Verification items for the finished model (mm, model axes). Round coordinates to 2 decimals unless told otherwise and drop trailing zeros. Order: outer loops, then holes, each group sorted by start corner. A loop starts at its lowest first (then second) coordinate and runs counter-clockwise, first axis right, second up. Notation, with made-up numbers: (20, 51.5) -> (35, 51.5) arc R23 cw to (35, 80.5) -> close; hole circle Ø3 at (-14, 2). An arc over 180 degrees is marked (long way). Put each result on its own line as item: value.
from build123d import *

# Parameters (mm, degrees)
SKETCH1_W             = 88.9
SKETCH1_H             = 66.04
SKETCH1_R             = 13.49375
BOSS_EXTRUDE1_DEPTH   = 6.35
F_6_CLEARANCE_HOLE1_D = 3.7973
F_6_CLEARANCE_HOLE2_D = 3.7973


with BuildPart() as part:
    # Sketch1 → Boss-Extrude1 (new body)
    with BuildSketch(Plane.XY):
        Rectangle(SKETCH1_W, SKETCH1_H)
        with Locations((0, -5.43814)):
            Circle(SKETCH1_R, mode=Mode.SUBTRACT)
    extrude(amount=BOSS_EXTRUDE1_DEPTH)

    # #6 Clearance Hole1 (through all)
    with Locations(Plane.XY.offset(6.35)):
        with Locations((-39.37, -26.67), (-29.21, -26.67), (29.21, -26.67), (39.37, -26.67)):
            Hole(F_6_CLEARANCE_HOLE1_D / 2)

    # #6 Clearance Hole2 (through all)
    with Locations(Plane(origin=(-39.37, 26.67, 6.35), x_dir=(1, 0, 0), z_dir=(0, 0, 1))):
        with Locations((0, 0), (10.16, 0), (68.58, 0), (78.74, 0)):
            Hole(F_6_CLEARANCE_HOLE2_D / 2)


solid = part.part
Item 1: Section check B-B on x = 0. Record the boundary of the cut face in (y, z), then the cut area to 3 significant figures.
Check sheet entries:
outline: (-33.02, 0) -> (-18.93, 0) -> (-18.93, 6.35) -> (-33.02, 6.35) -> close; (8.06, 0) -> (33.02, 0) -> (33.02, 6.35) -> (8.06, 6.35) -> close
area: 248 mm^2
Item 2: Material ranges on L1, parallel to Y at x = 39.37, z = 2.5; L2, parallel to Y at x = 0, z = 2.25; L3, parallel to Y at x = -9.5, z = 4.5, recorded low to high. Write a range as [from, to].
Check sheet entries:
L1: y = [-33.02, -28.57], [-24.77, 24.77], [28.57, 33.02]
L2: y = [-33.02, -18.93], [8.06, 33.02]
L3: y = [-33.02, -15.02], [4.14, 33.02]
Item 3: Section check A-A on y = -26.67. Record the boundary of the cut face in (x, z), then the cut area to 3 significant figures.
Check sheet entries:
outline: (-44.45, 0) -> (-41.27, 0) -> (-41.27, 6.35) -> (-44.45, 6.35) -> close; (-37.47, 0) -> (-31.11, 0) -> (-31.11, 6.35) -> (-37.47, 6.35) -> close; (-27.31, 0) -> (27.31, 0) -> (27.31, 6.35) -> (-27.31, 6.35) -> close; (31.11, 0) -> (37.47, 0) -> (37.47, 6.35) -> (31.11, 6.35) -> close; (41.27, 0) -> (44.45, 0) -> (44.45, 6.35) -> (41.27, 6.35) -> close
area: 468 mm^2
Item 4: Release check for a two-part mould opening along Y. For faces 1 (the cylindrical face through (37.616, -27.397, 3.131)), 2 (the flat face through (-1, -33.02, 3)), 3 (the flat face through (44.45, 0, 3)), 4 (the flat face through (-1, 33.02, 3)) record: +Y half, -Y half, draft (parallel to the pull), parting line (faces both ways), or undercut.
Check sheet entries:
face 1: undercut
face 2: -Y half
face 3: draft
face 4: +Y half
Item 5: Section check C-C on x = -29.21. Record the boundary of the cut face in (y, z), then the cut area to 3 significant figures.
Check sheet entries:
outline: (-33.02, 0) -> (-28.57, 0) -> (-28.57, 6.35) -> (-33.02, 6.35) -> close; (-24.77, 0) -> (24.77, 0) -> (24.77, 6.35) -> (-24.77, 6.35) -> close; (28.57, 0) -> (33.02, 0) -> (33.02, 6.35) -> (28.57, 6.35) -> close
area: 371 mm^2
Item 6: Section check D-D on z = 4. State how many separate pieces and enclosed holes the cut face has, then the cut area to 3 significant figures.
Check sheet entries:
separate pieces: 1
enclosed holes: 9
area: 5,210 mm^2
